from build123d import *

# Parameters (mm, degrees)
SKETCH1_W               = 30
SKETCH1_H               = 27
BOSS_EXTRUDE1_DEPTH     = 10
SKETCH2_R               = 1.115
CUT_EXTRUDE1_DEPTH      = 10
SKETCH2_4_R             = 5.329276436
SKETCH2_4_R_2           = 3.631824093
BOSS_EXTRUDE2_DEPTH     = 0.25
SKETCH2_5_R             = 0.25
CUT_EXTRUDE2_DEPTH      = 10
SKETCH4_R               = 0.65
CUT_EXTRUDE3_DEPTH      = 3
SKETCH5_W               = 14.6
SKETCH5_H               = 27
BOSS_EXTRUDE3_DEPTH     = 12
CUT_EXTRUDE4_DEPTH      = 12
CUT_EXTRUDE4_DEPTH_BACK = 15
SKETCH3_R               = 1.5
SKETCH7_R               = 4.2164
CUT_EXTRUDE5_DEPTH      = 9.8
SKETCH8_W               = 22
SKETCH8_H               = 27
CUT_EXTRUDE6_DEPTH      = 4
CHAMFER1_SIZE           = 4
SKETCH9_R               = 2
CUT_EXTRUDE7_DEPTH      = 2.5
CHAMFER2_SIZE           = 2.5
CHAMFER3_SIZE           = 0.3
CHAMFER4_SIZE           = 0.5


# Some blends are built 0.0001 mm under size
with BuildPart() as part:
    # Sketch1 → Boss-Extrude1 (new body)
    with BuildSketch(Plane.XY):
        with Locations((12, -10.5)):
            Rectangle(SKETCH1_W, SKETCH1_H)
    extrude(amount=-BOSS_EXTRUDE1_DEPTH)

    # Sketch2 → Cut-Extrude1 (cut)
    with BuildSketch(Plane.XY):
        with Locations((20.75, -1.75)):
            Circle(SKETCH2_R)
        with Locations((3.25, -19.25)):
            Circle(SKETCH2_R)
    extrude(amount=-CUT_EXTRUDE1_DEPTH, mode=Mode.SUBTRACT)

    # Sketch2<4> → Boss-Extrude2 (add)
    with BuildSketch(Plane.XY):
        with Locations((12, -10.5)):
            Circle(SKETCH2_4_R)
        with Locations((12, -10.5)):
            Circle(SKETCH2_4_R_2, mode=Mode.SUBTRACT)
    extrude(amount=BOSS_EXTRUDE2_DEPTH)

    # Sketch2<5> → Cut-Extrude2 (cut)
    with BuildSketch(Plane.XY):
        with Locations((12, -10.5)):
            Circle(SKETCH2_5_R)
    extrude(amount=-CUT_EXTRUDE2_DEPTH, mode=Mode.SUBTRACT)

    # Sketch4 → Cut-Extrude3 (cut)
    with BuildSketch(Plane.XY.offset(0.25)):
        with Locations((12, -6.055)):
            Circle(SKETCH4_R)
    extrude(amount=-CUT_EXTRUDE3_DEPTH, mode=Mode.SUBTRACT)

    # Sketch5 → Boss-Extrude3 (add)
    with BuildSketch(Plane.ZY.offset(3)):
        with Locations((-2.7, -10.5)):
            Rectangle(SKETCH5_W, SKETCH5_H)
    extrude(amount=BOSS_EXTRUDE3_DEPTH)

    # Sketch3 → Cut-Extrude4 (cut, two sides: drawn at the far end of the back side and taken through both)
    with BuildSketch(Plane.ZY.offset(3).offset(-CUT_EXTRUDE4_DEPTH_BACK)):
        with Locations((-2.7, -6.7)):
            Circle(SKETCH3_R)
    extrude(amount=CUT_EXTRUDE4_DEPTH + CUT_EXTRUDE4_DEPTH_BACK, mode=Mode.SUBTRACT)

    # Sketch7 → Cut-Extrude5 (cut)
    with BuildSketch(Plane.ZY.offset(15)):
        with Locations((-2.7, -6.7)):
            Circle(SKETCH7_R)
    extrude(amount=-CUT_EXTRUDE5_DEPTH, mode=Mode.SUBTRACT)

    # Sketch8 → Cut-Extrude6 (cut)
    with BuildSketch(Plane(origin=(0, 0, -10), x_dir=(-1, 0, 0), z_dir=(0, 0, -1))):
        with Locations((-12, -10.5)):
            Rectangle(SKETCH8_W, SKETCH8_H)
    extrude(amount=-CUT_EXTRUDE6_DEPTH, mode=Mode.SUBTRACT)

    # Chamfer1
    # the kernel refuses this chamfer: 4 mm, written as the material it adds along each edge
    with BuildSketch(Plane(origin=(1, 3, -6), x_dir=(0.9996219169112968, 0, 0.027495876610586275), z_dir=(0, -1, 0))) as chamfer1_piece_1_section:
        Polygon((CHAMFER1_SIZE * 0.999621916911, -CHAMFER1_SIZE * 0.0274958766106), (-CHAMFER1_SIZE * 0.0274958766106, -CHAMFER1_SIZE * 0.999621916911), (0, 0), align=None)
    chamfer1_piece_1 = extrude(amount=27, mode=Mode.PRIVATE)
    chamfer1_piece_1 = chamfer1_piece_1 - Plane(origin=(3.25, -19.25, -7.327035159), x_dir=(1, 0, 0), z_dir=(0, 0, 1)) * Cylinder(1.115, 70, mode=Mode.PRIVATE)
    chamfer1_piece_1 = split(chamfer1_piece_1, bisect_by=Plane(origin=(2.297726003, -10.22672805, -10), z_dir=(0, 0, 1)), keep=Keep.TOP, mode=Mode.PRIVATE)
    add(chamfer1_piece_1)
    with BuildSketch(Plane(origin=(23, -24, -6), x_dir=(0.027495876610586494, 0, -0.9996219169112968), z_dir=(0, 1, 0))) as chamfer1_piece_2_section:
        Polygon((CHAMFER1_SIZE * 0.999621916911, CHAMFER1_SIZE * 0.0274958766106), (-CHAMFER1_SIZE * 0.0274958766106, CHAMFER1_SIZE * 0.999621916911), (0, 0), align=None)
    chamfer1_piece_2 = extrude(amount=27, mode=Mode.PRIVATE)
    chamfer1_piece_2 = split(chamfer1_piece_2, bisect_by=Plane(origin=(21.702275046, -10.773273502, -10), z_dir=(0, 0, 1)), keep=Keep.TOP, mode=Mode.PRIVATE)
    chamfer1_piece_2 = chamfer1_piece_2 - Plane(origin=(20.75, -1.75, -7.327035315), x_dir=(1, 0, 0), z_dir=(0, 0, 1)) * Cylinder(1.115, 70, mode=Mode.PRIVATE)
    add(chamfer1_piece_2)

    # Sketch9 → Cut-Extrude7 (cut)
    with BuildSketch(Plane(origin=(0, 0, -6), x_dir=(-1, 0, 0), z_dir=(0, 0, -1))):
        with Locations((-12, -10.5)):
            Circle(SKETCH9_R)
    extrude(amount=-CUT_EXTRUDE7_DEPTH, mode=Mode.SUBTRACT)

    # Chamfer2
    chamfer2_edges = [part.edges().sort_by_distance(p)[0] for p in [
        (14, -10.5, -6),
    ]]
    chamfer(chamfer2_edges, length=CHAMFER2_SIZE - 0.0001)  # a hair under: the kernel refuses the full size

    # Chamfer3
    chamfer3_edges = [part.edges().sort_by_distance(p)[0] for p in [
        (3, -24, -8),
        (27, -10.5, -10),
        (-7, 3, -10),
        (-3, -24, 2.3),
        (-3, -10.5, 4.6),
        (-9, -24, 4.6),
        (-3, 3, 2.3),
        (-9, 3, 4.6),
        (-15, -10.5, -10),
        (-15, -24, -2.7),
        (-15, -10.5, 4.6),
        (-15, 3, -2.7),
        (12, 3, 0),
        (27, -10.5, 0),
        (12, -24, 0),
        (25, -24, -10),
        (25, 3, -10),
        (27, 3, -5),
        (27, -24, -5),
        (-7, -24, -10),
        (12, -24, -6),
        (12, 3, -6),
        (21, -24, -8),
        (21, 3, -8),
        (3, 3, -8),
    ]]
    chamfer(chamfer3_edges, length=CHAMFER3_SIZE)

    # Chamfer4
    chamfer4_edges = [part.edges().sort_by_distance(p)[0] for p in [
        (2.135, -19.25, 0),
        (19.635, -1.75, 0),
    ]]
    chamfer(chamfer4_edges, length=CHAMFER4_SIZE)


solid = part.part
Could you check a few things on this model? Use its own coordinates, in mm. A direction names the side the tool comes from. Give positions to 0.01 mm unless a question says otherwise; leave off trailing zeros. Loops run counter-clockwise (first coordinate to the right, second up) from the corner with the lowest first, then second, coordinate; pieces in that order, holes last. Notation, with made-up numbers: (31, 62.5) -> (44, 62.5) arc R9 cw to (44, 77.5) -> close; hole circle Ø3 at (61.5, -6). An arc over 180 degrees is marked (long way). Return JSON: item names as keys, results as strings.
Item 1: If we section it at B-B on z = 3.5: List the corners of the cut face in (x, y) for me, plus the area to 3 significant figures.
Geometry results:
{"outline": "(-15, -23.7) -> (-14.7, -24) -> (-3.3, -24) -> (-3, -23.7) -> (-3, 2.7) -> (-3.3, 3) -> (-14.7, 3) -> (-15, 2.7) -> close", "area": "324 mm²"}
Item 2: Which directions (+Z, -Z, +X, -X, +Y, -Y) give clear straight access to the entire face, cutting with the end or side of a thin tool? Please do faces 1 (the cylindrical face through (3.52, -5.213, -2.895)), 2 (the flat face through (14, -14, 0.25)), 3 (the flat face through (12, -16, 0)).
Geometry results:
{"face 1": "-X", "face 2": "+Z, +X, +Y, -Y", "face 3": "+Z"}
Item 3: If we section it at D-D on x = 20.75: List the corners of the cut face in (y, z) for me (3 decimals), plus the area to 4 significant figures.
Geometry results:
{"outline": "(-24, -7.326) -> (-23.7, -7.75) -> (-2.865, -7.75) -> (-2.865, -0.5) -> (-3.365, 0) -> (-23.7, 0) -> (-24, -0.3) -> close; (-0.635, -7.75) -> (2.7, -7.75) -> (3, -7.326) -> (3, -0.3) -> (2.7, 0) -> (-0.135, 0) -> (-0.635, -0.5) -> close", "area": "191.5 mm²"}
Item 4: If we section it at C-C on y = -16.5: List the corners of the cut face in (x, z) for me.
Geometry results:
{"outline": "(-15, -9.7) -> (-14.7, -10) -> (1, -10) -> (5, -6) -> (19, -6) -> (23, -10) -> (26.7, -10) -> (27, -9.7) -> (27, -0.3) -> (26.7, 0) -> (-3, 0) -> (-3, 4.3) -> (-3.3, 4.6) -> (-14.7, 4.6) -> (-15, 4.3) -> close"}
Item 5: We'd pull the mould along Y, two halves only. Please class faces 4 (the flat face through (-15, -13, -3)), 5 (the flat face through (12, -10, -3.5)), 6 (the flat face through (21.09, 2.85, -7.88)): +Y half, -Y half, draft (parallel to the pull), parting line (faces both ways), or undercut.
Geometry results:
{"face 4": "draft", "face 5": "undercut", "face 6": "+Y half"}
Item 6: I need wall thicknesses on L1, parallel to Z at x = 9.5, y = -6.75; L2, parallel to Y at x = 10, z = -4; L3, parallel to Z at x = 7.5, y = -6.7. Which ranges of each line are inside material? Lowest first, please. Write a range as from..to.
Geometry results:
{"L1": "z = -6..-4.2, -1.2..0.25", "L2": "y = -24..-12, -9..-7.45, -5.95..3", "L3": "z = -6..-4.2, -1.2..0"}
Item 7: I'm going to push flat-ended pins straight in: pin 1 (6 mm diameter, centred on x = 13, y = -10, fed in from +Z); pin 2 (7 mm diameter, centred on x = 12.5, y = -13.5, fed in from -Z); pin 3 (5 mm diameter, centred on x = 4.5, y = -10.5, fed in from -Z); pin 4 (1.3 mm diameter, centred on x = 3.25, y = -19.25, fed in from -Z). Where does each tip first touch, or does it pass through?
Geometry results:
{"pin 1": "stops at z = 0.25", "pin 2": "stops at z = -6", "pin 3": "stops at z = -9", "pin 4": "passes through"}
Item 8: If we section it at A-A on x = 6: List the corners of the cut face in (y, z) for me.
Geometry results:
{"outline": "(-24, -5.7) -> (-23.7, -6) -> (2.7, -6) -> (3, -5.7) -> (3, -0.3) -> (2.7, 0) -> (-23.7, 0) -> (-24, -0.3) -> close; hole circle Ø3 at (-6.7, -2.7)"}
